Could you check a few things on this drawing? It's one solid part, dimensions in mm from its lowest x, y, z. Coordinates: 2 decimals unless noted, no trailing zeros. Loops run counter-clockwise (first coordinate to the right, second up) from the corner with the lowest first, then second, coordinate; pieces in that order, holes last.
1) If I drill on line 1 along Y through (x, z) = (99, 2.5) (1 decimal); line 2 along X through (y, z) = (89.5, 1.25) (1 decimal); line 3 along Y through (x, z) = (77.5, 1.5), over which ranges is the centre line in solid material (lowest first)?
2) Imagine slicing it at D-D on x = 134.5. Please give me the cut outline in (y, z).
3) Imagine slicing it at B-B on y = 47.5. Please give me the cut outline in (x, z).
4) Imagine slicing it at A-A on z = 2. Please give me the cut outline in (x, y) (1 decimal).
5) Thinking about a two-plate mould opening in Z: for the marked faces 1 and 2, which applies, released by +Z, released by -Z, zero draft, split by the parting line, or undercut?
6) Will these pins go through, and if not, where does the flat tip stop? P1, Ø8, axis at x = 98, y = 124.5, coming from the +Z side; P2, Ø3, axis at x = 74, z = 1.5, coming from the +Y side (1 decimal).
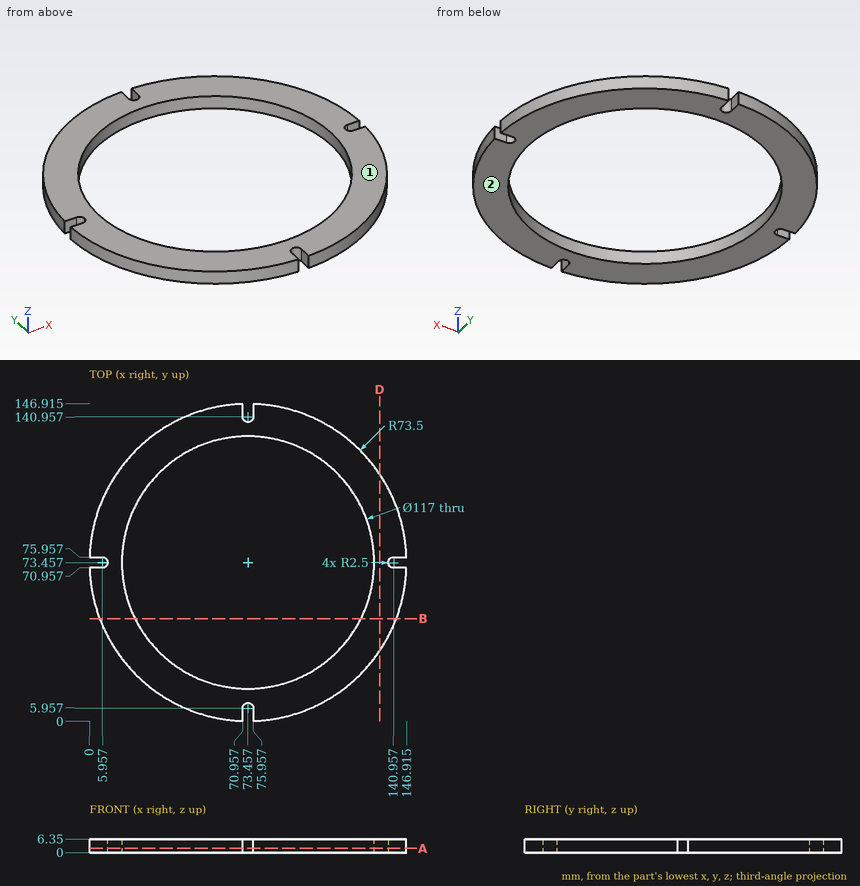
Filled in:
1. line 1: y = 4.5 to 20.8, 126.1 to 142.4
1. line 2: x = 1.7 to 17.2, 129.7 to 145.2
1. line 3: y = 0.07 to 15.1, 131.82 to 146.85
2. outline: (32.52, 0) - (114.4, 0) - (114.4, 6.35) - (32.52, 6.35) - close
3. outline: (4.69, 0) - (21.03, 0) - (21.03, 6.35) - (4.69, 6.35) - close; (125.88, 0) - (142.22, 0) - (142.22, 6.35) - (125.88, 6.35) - close
4. outline: (0, 71) arc R73.5 ccw to (71, 0) - (71, 6) arc R2.5 cw to (76, 6) - (76, 0) arc R73.5 ccw to (146.9, 71) - (141, 71) arc R2.5 cw to (141, 76) - (146.9, 76) arc R73.5 ccw to (76, 146.9) - (76, 141) arc R2.5 cw to (71, 141) - (71, 146.9) arc R73.5 ccw to (0, 76) - (6, 76) arc R2.5 cw to (6, 71) - close; hole circle Ø117 at (73.5, 73.5)
5. face 1: released by +Z
5. face 2: released by -Z
6. P1: stops at z = 6.35
6. P2: stops at y = 139.5
